Verification items for the finished model (mm, model axes). Coordinates: 2 decimals unless noted, no trailing zeros. Order: outer loops, then holes, each group sorted by start corner. A loop starts at its lowest first (then second) coordinate and runs counter-clockwise, first axis right, second up. Notation, with made-up numbers: (80, 25) -> (118, 25) arc R3 ccw to (118, 29) -> close; hole circle Ø2 at (-36, 25.5). An arc over 180 degrees is marked (long way). Write item = value, one per line. Start each with the question number.
1. Cross-section at B-B on y = -12.5. Record the cut outline in (x, z).
2. Thickness scan on line 1 along X through (y, z) = (-18, -0.05); line 2 along Y through (x, z) = (37, -1.15). Record the ranges inside material, lowest first. Write a range as from..to.
3. Cross-section at A-A on x = 95. Record the cut outline in (y, z).
4. Cross-section at C-C on z = -0.9. Record the cut outline in (x, y).
Autodesk Inventor part; units mm, degrees
ref_plane "YZ Plane" through (0, 0, 0) normal (1, 0, 0) x (0, 1, 0)
ref_plane "XZ Plane" through (0, 0, 0) normal (0, 1, 0) x (-1, 0, 0)
ref_plane "XY Plane" through (0, 0, 0) normal (0, 0, 1) x (1, 0, 0)
sketch "Sketch1" plane through (0, 0, 0) normal (0, 0, 1) x (1, 0, 0)
  line L0 (109.2, 0) -> (109.2, -84)
  line L1 (0, -84) -> (0, 0)
  line L2 (0, -84) -> (109.2, -84)
  line L3 (109.2, -84) -> (109.2, 0)
  line L4 (109.2, 0) -> (0, 0)
  line L5 (0, 0) -> (0, -84)
  line L6 (-11.4, 31.9489) -> (120.6, 31.9489)
  line L7 (120.6, 31.9489) -> (120.6, -96.5511)
  line L8 (120.6, -96.5511) -> (-11.4, -96.5511)
  line L9 (-11.4, -96.5511) -> (-11.4, 31.9489)
  line L10 (117.1, 20.1989) -> (-7.9, 20.1989)
  line L11 (-7.9, 20.1989) -> (-7.9, -84.8011)
  line L12 (-7.9, -84.8011) -> (117.1, -84.8011)
  line L13 (117.1, -84.8011) -> (117.1, 20.1989)
  line L14 (-7.9, -84.8011) -> (-7.9, -96.5511)
  line L15 (-7.9, 20.1989) -> (-7.9, 31.9489)
  line L16 (109.2, -42) -> (117.1, -42)
  line L17 (0, -42) -> (-7.9, -42)
  line L18 (120.6, -32.3011) -> (117.1, -32.3011)
  line L19 (-7.9, -32.3011) -> (-11.4, -32.3011)
  dimension "d0" = 128.5
  dimension "d1" = 105
  dimension "d3" = 125
  dimension "d4" = 132
extrude "Extrusion1" add sketch "Sketch1" against normal blind 1.6 contours L4 L1 L17 L11 L10 L13 L16 L0 | L16 L13 L12 L11 L17 L1 L2 L0 | L13 L18 L7 L8 L14 L12 | L13 L10 L15 L6 L7 L18 | L11 L14 L8 L9 L19 | L19 L9 L6 L15 L11
properties part number "Frontpanel"
Worked out:
q1.outline = (-11.4, -1.6) -> (0, -1.6) -> (0, 0) -> (-11.4, 0) -> close; (109.2, -1.6) -> (120.6, -1.6) -> (120.6, 0) -> (109.2, 0) -> close
q2.line_1 = -11.4..0, 109.2..120.6
q2.line_2 = -96.55..-84, 0..31.95
q3.outline = (-96.55, -1.6) -> (-84, -1.6) -> (-84, 0) -> (-96.55, 0) -> close; (0, -1.6) -> (31.95, -1.6) -> (31.95, 0) -> (0, 0) -> close
q4.outline = (-11.4, -96.55) -> (120.6, -96.55) -> (120.6, 31.95) -> (-11.4, 31.95) -> close; hole (0, -84) -> (109.2, -84) -> (109.2, 0) -> (0, 0) -> close
